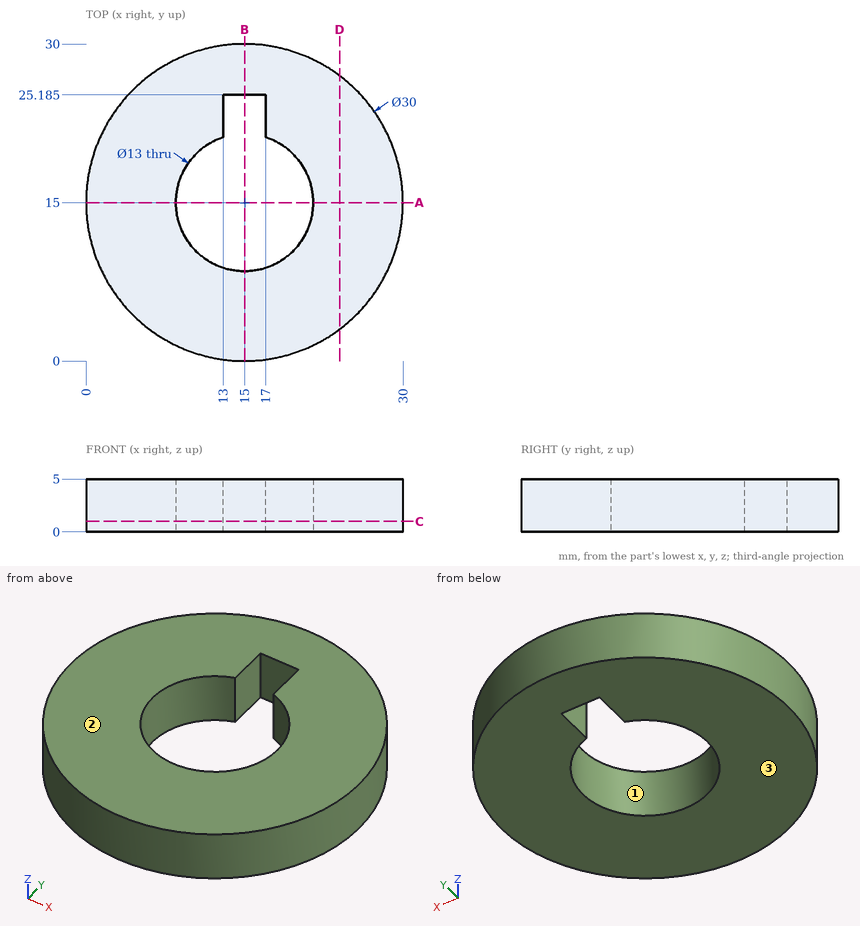
Geometry check sheet. Reference: drawing and pictorial views, mm from the part's lowest x, y, z. Coordinates: 2 decimals unless noted, no trailing zeros. Order: outer loops, then holes, each group sorted by start corner. A loop starts at its lowest first (then second) coordinate and runs counter-clockwise, first axis right, second up.
1. Scan lines: line 1 (X direction, y = 14.75, z = 4.3) (1 decimal); line 2 (Y direction, x = 15, z = 4.05) (1 decimal); line 3 (X direction, y = 22.5, z = 1.65). Record each from-to range of solid material in increasing order.
Results found:
line 1: x = 0 to 8.5, 21.5 to 30
line 2: y = 0 to 8.5, 25.2 to 30
line 3: x = 2.01 to 13, 17 to 27.99
2. Sectioned sample at A-A, the plane y = 15. Record the cut outline in (x, z), and give its area (3 significant figures).
Results found:
outline: (0, 0) - (8.5, 0) - (8.5, 5) - (0, 5) - close; (21.5, 0) - (30, 0) - (30, 5) - (21.5, 5) - close
area: 85.0 mm2
3. Sectioned sample at C-C, the plane z = 1. Record the cut outline in (x, y) (1 decimal).
Results found:
outline: circle Ø30 at (15, 15); hole (13, 21.2) arc R6.5 ccw (long way) to (17, 21.2) - (17, 25.2) - (13, 25.2) - close
4. Go/stop test with flat-tipped pins: pin 1 Ø3 at (y, z) = (23, 2) entering from -X; pin 2 Ø1.5 at (y, z) = (27, 3.5) entering from -X; pin 3 Ø3 at (x, z) = (6.5, 1) entering from +Y; pin 4 Ø8 at (x, y) = (15, 17.5) entering from +Z. Record where each tip stops, or that it passes through.
Results found:
pin 1: stops at x = 1.48
pin 2: stops at x = 5.08
pin 3: stops at y = 28.27
pin 4: passes through
5. Sectioned sample at B-B, the plane x = 15. Record the cut outline in (y, z) (1 decimal).
Results found:
outline: (0, 0) - (8.5, 0) - (8.5, 5) - (0, 5) - close; (25.2, 0) - (30, 0) - (30, 5) - (25.2, 5) - close
6. Sectioned sample at D-D, the plane x = 24. Record the cut outline in (y, z).
Results found:
outline: (3, 0) - (27, 0) - (27, 5) - (3, 5) - close
7. Release check for a two-part mould opening along Z. For the marked faces 1, 2 and 3 record: +Z half, -Z half, draft (parallel to the pull), parting line (faces both ways), or undercut.
Results found:
face 1: draft
face 2: +Z half
face 3: -Z half
